Source: three-view drawing plus pictorial views. Frame: mm from the lowest corner of the part. Give positions to 0.01 mm unless a question says otherwise; leave off trailing zeros. Order: outer loops, then holes, each group sorted by start corner. A loop starts at its lowest first (then second) coordinate and runs counter-clockwise, first axis right, second up. Notation, with made-up numbers: (-39, 89) -> (4, 89) arc R19 ccw to (4, 101) -> close; hole circle Ø8 at (67.25, 66.5). An arc over 180 degrees is marked (long way). Answer in a Markdown table with one row per item. Add a question column.
Q1. Cut plane C-C on z = 11.25. Return the cut outline in (x, y).
Q2. Line query: line 1 along X through (y, z) = (4.5, 2) (1 decimal); line 2 along Z through (x, y) = (5.25, 0.5) (1 decimal); line 3 along X through (y, z) = (1, 1.25). Output: solid intervals per line, ascending. Write a range as from..to.
Q3. Cut plane B-B on z = 18.75. Return the cut outline in (x, y).
Q4. Contact query for a flat-ended pin moving along its axis: P1, Ø6, axis at y = 8.5, z = 4.5, coming from the -X side. Output: stop coordinate, or through.
Q5. Cut plane A-A on y = 4. Return the cut outline in (x, z) (1 decimal).
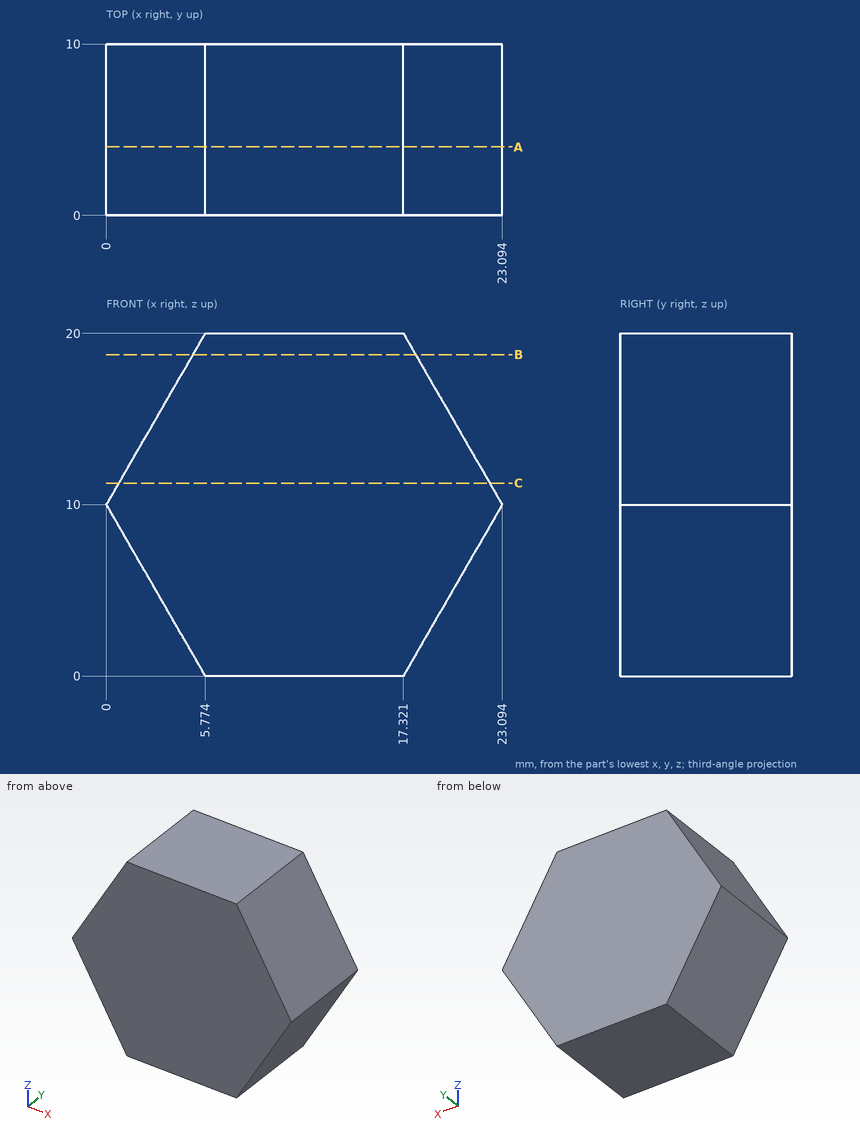
Completed:
| question | item | result |
|---|---|---|
| 1 | outline | (0.72, 0) -> (22.37, 0) -> (22.37, 10) -> (0.72, 10) -> close |
| 2 | line 1 | x = 4.6..18.5 |
| 2 | line 2 | z = 0.9..19.1 |
| 2 | line 3 | x = 5.05..18.04 |
| 3 | outline | (5.05, 0) -> (18.04, 0) -> (18.04, 10) -> (5.05, 10) -> close |
| 4 | P1 | stops at x = 1.44 |
| 5 | outline | (0, 10) -> (5.8, 0) -> (17.3, 0) -> (23.1, 10) -> (17.3, 20) -> (5.8, 20) -> close |
